Geometry check sheet. Reference: drawing and pictorial views, mm from the part's lowest x, y, z. A direction names the side the tool comes from. Coordinates: 2 decimals unless noted, no trailing zeros. Loops run counter-clockwise (first coordinate to the right, second up) from the corner with the lowest first, then second, coordinate; pieces in that order, holes last. Notation, with made-up numbers: (31, 24) - (64, 24) arc R23 cw to (64, 48) - close; hole circle Ø8 at (19, -11.75). An arc over 180 degrees is marked (long way). Use a Markdown table: item, result. Add a question column.
1) Sectioned sample at B-B, the plane z = 4.75. Enter the section's corners in (x, y).
2) Sectioned sample at A-A, the plane y = 2.25. Enter the section's corners in (x, z).
3) Sectioned sample at C-C, the plane x = 21.25. Enter the section's corners in (y, z).
4) Go/stop test with flat-tipped pins: P1, Ø8, axis at y = 14.5, z = 3, coming from the -X side; P2, Ø2.5, axis at y = 13.5, z = 18, coming from the +X side; P3, Ø6, axis at x = 24.5, y = 3, coming from the +Z side. Record where each tip stops, or that it passes through.
5) Tool access check on the marked faces 1, 2 and 3. Record the directions out of +Z, -Z, +X, -X, +Y, -Y that give a thin tool (end or side, any length) a straight path to the whole face; none if there is none.
6) Thickness scan on line 1 (X direction, y = 17, z = 5.5); line 2 (X direction, y = 14.5, z = 16); line 3 (Z direction, x = 6.5, y = 12). Record the ranges inside material, lowest first.
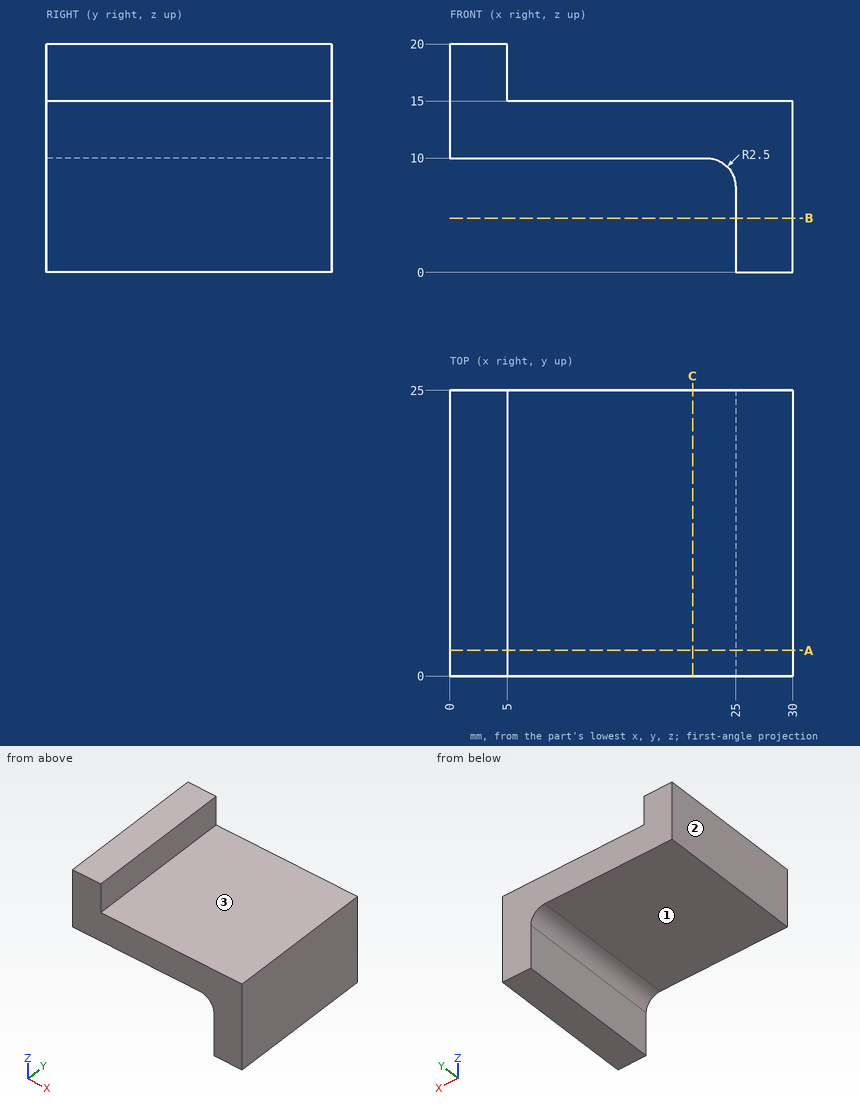
Solved:
| question | item | result |
|---|---|---|
| 1 | outline | (25, 0) - (30, 0) - (30, 25) - (25, 25) - close |
| 2 | outline | (0, 10) - (22.5, 10) arc R2.5 cw to (25, 7.5) - (25, 0) - (30, 0) - (30, 15) - (5, 15) - (5, 20) - (0, 20) - close |
| 3 | outline | (0, 10) - (25, 10) - (25, 15) - (0, 15) - close |
| 4 | P1 | stops at x = 25 |
| 4 | P2 | stops at x = 5 |
| 4 | P3 | stops at z = 15 |
| 5 | face 1 | -Z, -X, +Y, -Y |
| 5 | face 2 | +Z, -Z, -X, +Y, -Y |
| 5 | face 3 | +Z, +X, +Y, -Y |
| 6 | line 1 | x = 25 to 30 |
| 6 | line 2 | x = 0 to 5 |
| 6 | line 3 | z = 10 to 15 |
